```python
from build123d import *

# Parameters (mm, degrees)
ESBO_O1_W                = 19.05
ESBO_O1_H                = 360
RESSALTO_EXTRUS_O1_DEPTH = 9.525
ESBO_O3_R                = 2.5
CORTE_EXTRUS_O1_DEPTH    = 181.503327532


with BuildPart() as part:
    # Esboço1 → Ressalto-extrusão1 (new body)
    with BuildSketch(Plane.XY):
        Rectangle(ESBO_O1_W, ESBO_O1_H)
    extrude(amount=RESSALTO_EXTRUS_O1_DEPTH)

    # Esboço3 → Corte-extrusão1 (cut, through all)
    with BuildSketch(Plane.XY.offset(9.525)):
        with Locations((0, -173.65)):
            Circle(ESBO_O3_R)
    extrude(amount=-CORTE_EXTRUS_O1_DEPTH, mode=Mode.SUBTRACT)

    # Esboço5 → Rebaixo para parafuso com cabeça panela de M51 (revolve, cut)
    with BuildSketch(Plane(origin=(0, -173.65, 9.525), x_dir=(0, -1, 0), z_dir=(1, 0, 0))):
        Polygon((0, 0), (0, 9.525), (2.75, 9.525), (2.75, 3.7), (5.5, 3.7), (5.5, 0.025), (5.525, 0), align=None)
    revolve(axis=Axis((0, -173.65, 15.875), (0, 0, -1)), mode=Mode.SUBTRACT)


solid = part.part
```
The listing builds one solid part. Answer for the finished solid, in the listing's coordinates (mm). A direction names the side the tool comes from. Give positions to 0.01 mm unless a question says otherwise; leave off trailing zeros. Put each result on its own line as item: value. Start each with the question number.
Item 1: Find the intervals of material crossed by line 1 along Y through (x, z) = (0, 7.4); line 2 along X through (y, z) = (-173.65, 3.9) (3 decimals); line 3 along X through (y, z) = (-173.65, 7.85) (3 decimals), in increasing order.
Item 2: Flat-ended cylindrical pins translate along their axes: P1, Ø9, axis at x = -2, y = -172, coming from the +Z side (3 decimals); P2, Ø7, axis at x = 0, y = -173.65, coming from the +Z side (3 decimals). Find the tip coordinate at first contact, or state that the pin passes through.
Item 3: Which of the six approach directions +Z, -Z, +X, -X, +Y, -Y give full straight-line access (tool end or side, diameter ignored) to faces 1 (the face through (-0.242, -168.155, 7.688)), 2 (the face through (-9.525, -3, 5))?
Item 4: For a pull along Y with two mould halves and no side action, classify faces 3 (the face through (0, -180, 5)), 4 (the face through (0, 3, 0)), 5 (the face through (-0.83, -176.27, 2.95)) as +Y half, -Y half, draft (parallel to the pull), parting line (faces both ways), or undercut.
Answer key:
1. line 1: y = -180 to -179.15, -168.15 to 180
1. line 2: x = -9.525 to -2.75, 2.75 to 9.525
1. line 3: x = -9.525 to -5.5, 5.5 to 9.525
2. P1: stops at z = 9.525
2. P2: stops at z = 5.825
3. face 1: +Z
3. face 2: +Z, -Z, -X, +Y, -Y
4. face 3: -Y half
4. face 4: draft
4. face 5: undercut
